The model under review builds one solid part; all positions refer to its coordinate system, in mm. A direction names the side the tool comes from. Coordinates: 2 decimals unless noted, no trailing zeros. Order: outer loops, then holes, each group sorted by start corner. A loop starts at its lowest first (then second) coordinate and runs counter-clockwise, first axis right, second up. Notation, with made-up numbers: (73, 35) -> (116, 35) arc R9 ccw to (116, 41) -> close; hole circle Ø10 at (69, 70). An arc over 180 degrees is marked (long way). Use one line per item in the form item = value.
from build123d import *

# Parameters (mm, degrees)
SKETCH046_W     = 42
SKETCH046_H     = 42
PAD022_DEPTH    = 14
SKETCH047_R     = 7
PAD023_DEPTH    = 2.5
SKETCH048_R     = 3
HOLE_DEPTH      = 0.5
HOLE_TIPS_R     = 3
SKETCH049_W     = 23.5
SKETCH049_H     = 5.5
POCKET008_DEPTH = 5


with BuildPart() as part:
    # Sketch046 → Pad022 (new body)
    with BuildSketch(Plane.XZ):
        with Locations((8.147526, -9.378734)):
            Rectangle(SKETCH046_W, SKETCH046_H)
    extrude(amount=PAD022_DEPTH)

    # Sketch047 (on Face5 of Pad022) → Pad023 (join)
    with BuildSketch(Plane(origin=(0, 0, 0), x_dir=(1, 0, 0), z_dir=(0, 1, 0))):
        with Locations((8.142856, 9.219142)):
            Circle(SKETCH047_R)
    extrude(amount=PAD023_DEPTH)

    # Sketch048 (on Face8 of Pad023) → Hole (cut)
    with BuildSketch(Plane(origin=(0, 2.5, 0), x_dir=(1, 0, 0), z_dir=(0, 1, 0))):
        with Locations((8.27745, 9.219093)):
            Circle(SKETCH048_R)
    extrude(amount=-HOLE_DEPTH, mode=Mode.SUBTRACT)

    # Hole tips → Hole tip 1 section 0
    with BuildSketch(Plane(origin=(0, 2, 0), x_dir=(1, 0, 0), z_dir=(0, 1, 0)), mode=Mode.PRIVATE) as hole_tip_1_s0:
        with Locations((8.27745, 9.219093)):
            Circle(HOLE_TIPS_R)
    loft([hole_tip_1_s0.sketch, Vertex(8.27745, 0.197418, -9.219093)], mode=Mode.SUBTRACT)

    # Sketch049 (on Face5 of Hole) → Pocket008 (cut)
    with BuildSketch(Plane.XZ.offset(14)):
        with Locations((8.721823, -22.801634)):
            Rectangle(SKETCH049_W, SKETCH049_H)
    extrude(amount=-POCKET008_DEPTH, mode=Mode.SUBTRACT)


with BuildPart() as part_1:
    # Body007 placement: moved
    add(part.part.moved(Location((-10, 80, 143.5))))


solid = part_1.part
Item 1: We need section C-C (x = -10.5). Write out the cut boundary in (y, z).
Results found:
outline = (66, 113.12) -> (80, 113.12) -> (80, 155.12) -> (66, 155.12) -> (66, 123.45) -> (71, 123.45) -> (71, 117.95) -> (66, 117.95) -> close
Item 2: We need section A-A (y = 70.5). Write out the cut boundary in (x, z), plus the area to 3 significant figures.
Results found:
outline = (-22.85, 113.12) -> (19.15, 113.12) -> (19.15, 155.12) -> (-22.85, 155.12) -> close; hole (-13.03, 117.95) -> (10.47, 117.95) -> (10.47, 123.45) -> (-13.03, 123.45) -> close
area = 1,630 mm²
Item 3: To check wall thickness, follow L1, parallel to Z at x = -1, y = 69.25; L2, parallel to Y at x = 7, z = 128; L3, parallel to Y at x = -6.5, z = 120. State the ranges of each line that lie inside material, in increasing order. Write a range as from..to.
Results found:
L1 = 113.12..117.95, 123.45..155.12
L2 = 66..80
L3 = 71..80
Item 4: We need section D-D (x = 13.5). Write out the cut boundary in (y, z), plus the area to 3 significant figures.
Results found:
outline = (66, 113.12) -> (80, 113.12) -> (80, 155.12) -> (66, 155.12) -> close
area = 588 mm²
Item 5: We need section B-B (z = 119). Write out the cut boundary in (x, y), plus the area to 4 significant figures.
Results found:
outline = (-22.85, 66) -> (-13.03, 66) -> (-13.03, 71) -> (10.47, 71) -> (10.47, 66) -> (19.15, 66) -> (19.15, 80) -> (-22.85, 80) -> close
area = 470.5 mm²
Item 6: Draft analysis for pull direction X (two halves, no side actions). For faces 4 (the face through (10.472, 68, 121)), 5 (the face through (-2.77, 81.23, 127.34)), 6 (the face through (0, 82.5, 137)), state which applies: released by +X, released by -X, zero draft, split by the parting line, or undercut.
Results found:
face_4 = undercut
face_5 = split by the parting line
face_6 = zero draft
Item 7: Tool access review of faces 1 (the face through (-13.028, 68, 121)), 2 (the face through (-2, 80, 125)), 3 (the face through (-2, 73, 155.121)): name each direction out of +Z, -Z, +X, -X, +Y, -Y from which nothing blocks a thin tool from reaching the whole face with its end or side.
Results found:
face_1 = -Y
face_2 = +Y
face_3 = +Z, +X, -X, +Y, -Y
